```python
from build123d import *

# Parameters (mm, degrees)
F1_DEPTH = 10
F2_R     = 5
F3_R     = 1


with BuildPart() as f1:
    # F0 (on Top) → F1 (new body)
    with BuildSketch(Plane.XY):
        Polygon((-8, 182), (-6, 182), (-6, 200), (0, 200), (0, 0), (86, 0), (86, 20), (84, 20), (84, 2), (44, 2), (44, 4), (42, 4), (42, 2), (2, 2), (2, 202), (-8, 202), align=None)
    extrude(amount=F1_DEPTH)

    # F2
    f2_edges = [f1.edges().sort_by_distance(p)[0] for p in [
        (2, 2, 5),
        (84, 2, 5),
    ]]
    fillet(f2_edges, radius=F2_R)

    # F3
    f3_edges = [f1.edges().sort_by_distance(p)[0] for p in [
        (-6, 200, 5),
        (0, 200, 5),
    ]]
    fillet(f3_edges, radius=F3_R)


solid = f1.part
```
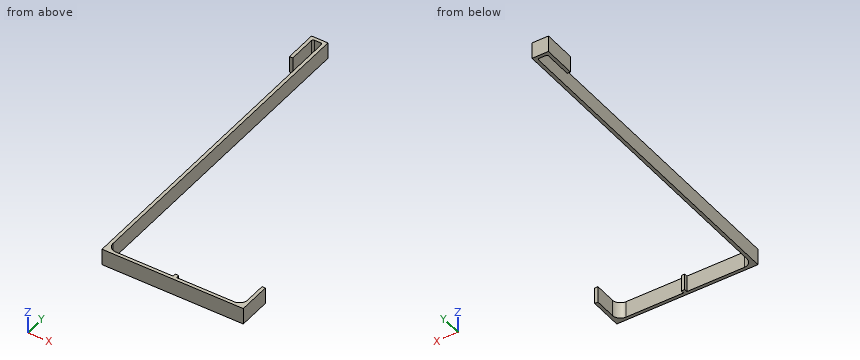
Work out the finished part from the listing and answer in its coordinate system (mm). Coordinates: 2 decimals unless noted, no trailing zeros. Write each loop counter-clockwise with the first axis right and the second up, starting at its lowest first coordinate (ties: lowest second). Pieces come first, ordered by that corner, then holes.
Q1. Find the intervals of material crossed by line 1 (Y direction, x = 63, z = 5.5); line 2 (Y direction, x = -2, z = 3.5), in increasing order.
Q2. A cutting plane is placed at A-A, the plane z = 5. Give the vertices of the cut face in (x, y).
Q3. Each of these flat-tipped pins is pushed along its axis until it touches: pin 1 Ø1 at (x, z) = (43, 3) entering from +Y; pin 2 Ø1 at (y, z) = (75.5, 4.5) entering from -X; pin 3 Ø5 at (y, z) = (127.5, 5.5) entering from +X. Where does it stop, or does it pass through?
Q4. A cutting plane is placed at B-B, the plane y = 23. Give the vertices of the cut face in (x, z).
Findings below:
1. line 1: y = 0 to 2
1. line 2: y = 200 to 202
2. outline: (-8, 182) - (-6, 182) - (-6, 199) arc R1 cw to (-5, 200) - (-1, 200) arc R1 cw to (0, 199) - (0, 0) - (86, 0) - (86, 20) - (84, 20) - (84, 7) arc R5 cw to (79, 2) - (44, 2) - (44, 4) - (42, 4) - (42, 2) - (7, 2) arc R5 cw to (2, 7) - (2, 202) - (-8, 202) - close
3. pin 1: stops at y = 4
3. pin 2: stops at x = 0
3. pin 3: stops at x = 2
4. outline: (0, 0) - (2, 0) - (2, 10) - (0, 10) - close
